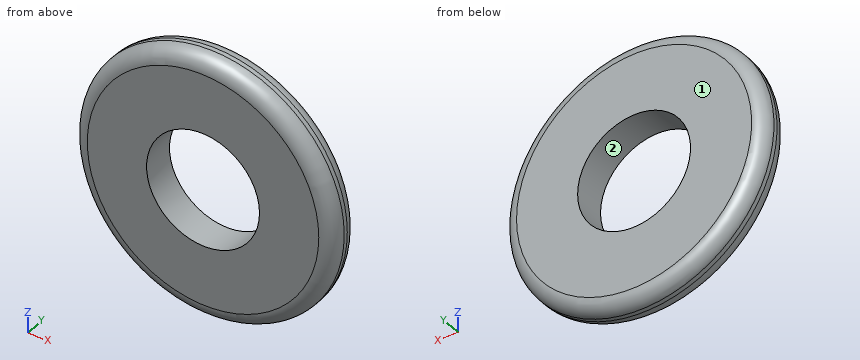
```python
from build123d import *

# Parameters (mm, degrees)
F1_R     = 60.8108481728
F3_DEPTH = 15.0508303195
F4_R     = 26.2822858087
F5_DEPTH = 160.9226148576
F6_R     = 6.0899953587
F7_R     = 6.9381681598


with BuildPart() as f3:
    # F1 (on face) → F3 (new body)
    with BuildSketch(Plane.XZ):
        Circle(F1_R)
    extrude(amount=F3_DEPTH)

    # F4 (on face) → F5 (cut)
    with BuildSketch(Plane.XZ):
        Circle(F4_R)
    extrude(amount=F5_DEPTH, mode=Mode.SUBTRACT)

    # F6
    f6_edges = [f3.edges().sort_by_distance(p)[0] for p in [
        (-60.810848, 0, 0),
    ]]
    fillet(f6_edges, radius=F6_R)

    # F7
    f7_edges = [f3.edges().sort_by_distance(p)[0] for p in [
        (-60.810848, -15.05083, 0),
    ]]
    fillet(f7_edges, radius=F7_R)


solid = f3.part
```
Read the model definition and answer for the solid it produces. Units are mm, in the model's axes. Face numbers are marked on the shaded views. Give positions to 0.01 mm unless a question says otherwise; leave off trailing zeros. Loops run counter-clockwise (first coordinate to the right, second up) from the corner with the lowest first, then second, coordinate; pieces in that order, holes last.
Item 1: The part is cut by section D-D (y = -10). Write down the section's boundary in (x, z), and give its area (3 significant figures).
Item 2: Each of these flat-tipped pins is pushed along its axis until it touches: pin 1 Ø1.5 at (y, z) = (-13, 0) entering from -X; pin 2 Ø2 at (y, z) = (-12, -38.5) entering from -X; pin 3 Ø5 at (y, z) = (-2, -44.5) entering from -X. Where does it stop, or does it pass through?
Item 3: The part is cut by section A-A (z = 0). Write down the section's boundary in (x, y).
Item 4: The mould has two halves that part along Z. Classify the marked faces 1 and 2: released by +Z, released by -Z, zero draft, split by the parting line, or undercut.
Item 5: Find the intervals of material crossed by line 1 along Z through (x, y) = (0, -5.75); line 2 along Z through (x, y) = (0, -4.25); line 3 along X through (y, z) = (-8.5, -10), in increasing order.
Item 6: The part is cut by section B-B (x = 0). Write down the section's boundary in (y, z).
Item 7: The part is cut by section C-C (y = -1.5). Write down the section's boundary in (x, z), and give its area (3 significant figures).
Taken from the geometry:
1. outline: circle Ø121.1 at (0, 0); hole circle Ø52.56 at (0, 0)
1. area: 9,350 mm2
2. pin 1: stops at x = -59.44
2. pin 2: stops at x = -46.66
2. pin 3: stops at x = -42.68
3. outline: (-60.81, -8.11) arc R6.94 ccw to (-53.87, -15.05) - (-26.28, -15.05) - (-26.28, 0) - (-54.72, 0) arc R6.09 ccw to (-60.81, -6.09) - close; (26.28, -15.05) - (53.87, -15.05) arc R6.94 ccw to (60.81, -8.11) - (60.81, -6.09) arc R6.09 ccw to (54.72, 0) - (26.28, 0) - close
4. face 1: zero draft
4. face 2: undercut
5. line 1: z = -60.8 to -26.28, 26.28 to 60.8
5. line 2: z = -60.53 to -26.28, 26.28 to 60.53
5. line 3: x = -59.97 to -24.31, 24.31 to 59.97
6. outline: (-15.05, -53.87) arc R6.94 ccw to (-8.11, -60.81) - (-6.09, -60.81) arc R6.09 ccw to (0, -54.72) - (0, -26.28) - (-15.05, -26.28) - close; (-15.05, 26.28) - (0, 26.28) - (0, 54.72) arc R6.09 ccw to (-6.09, 60.81) - (-8.11, 60.81) arc R6.94 ccw to (-15.05, 53.87) - close
7. outline: circle Ø117.45 at (0, 0); hole circle Ø52.56 at (0, 0)
7. area: 8,660 mm2
